Autodesk Inventor part; units mm, degrees
ref_plane "YZ Plane" through (0, 0, 0) normal (1, 0, 0) x (0, 1, 0)
ref_plane "XZ Plane" through (0, 0, 0) normal (0, 1, 0) x (-1, 0, 0)
ref_plane "XY Plane" through (0, 0, 0) normal (0, 0, 1) x (1, 0, 0)
sketch "Esquisse5" plane through (0, 0, 0) normal (0, 0, 1) x (1, 0, 0)
  line L0 (0, 0) -> (20, 0)
  line L1 (20, 0) -> (20, 30)
  line L2 (20, 30) -> (0, 30)
  line L3 (0, 30) -> (0, 0)
  line L4 (10, 0) -> (10, 30) construction
  circle A0 centre (10, 9) radius 2.15
  circle A1 centre (10, 15) radius 2.15
  circle A2 centre (10, 21) radius 2.15
  line L5 (10, 15) -> (20, 15) construction
  circle A3 centre (16, 15) radius 2.15
  circle A4 centre (4, 15) radius 2.15
  circle A5 centre (10, 15) radius 2.15
  dimension "d61" = 20
  dimension "d62" = 30
  dimension "d64" = 4.3
  dimension "d67" = 6
  dimension "d74" = 6
  dimension "d77" = 6
extrude "Extrusion5" add sketch "Esquisse5" along normal blind 2.2
sketch "Esquisse9" plane through (0, 0, 2.2) normal (0, 0, 1) x (1, 0, 0)
  line L0 (20, 0) -> (20, 30) construction
  line L1 (0, 30) -> (0, 0) construction
  line L2 (0, 30) -> (20, 30)
  line L3 (20, 30) -> (20, 27)
  line L4 (20, 27) -> (0, 27)
  line L5 (0, 27) -> (0, 30)
  line L6 (0, 15) -> (20, 15) construction
  line L7 (20, 0) -> (0, 0) construction
  line L8 (0, 0) -> (20, 0)
  line L9 (20, 0) -> (20, 3)
  line L10 (20, 3) -> (0, 3)
  line L11 (0, 3) -> (0, 0)
  dimension "d102" = 3
extrude "Extrusion9" add sketch "Esquisse9" along normal blind 10
sketch "Esquisse10" plane through (0, 0, 0) normal (0, -1, 0) x (1, 0, 0)
  line L0 (0, 0) -> (20, 0) construction
  line L1 (20, 0) -> (20, 12.2) construction
  line L2 (0, 12.2) -> (20, 12.2) construction
  line L3 (10, 12.2) -> (10, 0) construction
  circle A0 centre (10, 8.2) radius 2.15
  line L4 (10, 8.2) -> (20, 8.2) construction
  circle A1 centre (16, 8.2) radius 2.15
  circle A2 centre (4, 8.2) radius 2.15
  circle A3 centre (10, 8.2) radius 2.15
  dimension "d105" = 4
  dimension "d106" = 4.3
  dimension "d109" = 6
  dimension "d112" = 6
extrude "Extrusion10" cut sketch "Esquisse10" against normal through all
fillet "Congé6" radius 2 8 edges at (10, 0, 0) (10, 3, 2.2) (10, 27, 2.2) (0, 28.5, 12.2) (20, 28.5, 12.2) (20, 1.5, 12.2) (0, 1.5, 12.2) (10, 30, 0)
equation "\"d64\" = Holes"
equation "\"d80\" = Depth"
equation "\"d106\" = Holes"
equation "\"Depth\" = 2.2"
equation "\"Holes\" = 4.3"
equation "\"Height\" = 0"
equation "\"Rounding\" = 7"
properties part number "Pantilt"
Could you check a few things on this model? Use its own coordinates, in mm. A direction names the side the tool comes from. Give positions to 0.01 mm unless a question says otherwise; leave off trailing zeros. Loops run counter-clockwise (first coordinate to the right, second up) from the corner with the lowest first, then second, coordinate; pieces in that order, holes last. Notation, with made-up numbers: (-39, 69) -> (-18, 69) arc R27 cw to (-18, 95) -> close; hole circle Ø3 at (28.25, -23). An arc over 180 degrees is marked (long way). Return JSON: item names as keys, results as strings.
Item 1: If we section it at A-A on z = 8.2: Count the separate pieces of the cut face and the enclosed holes in it, plus the area to 3 significant figures.
Geometry results:
{"separate pieces": "8", "enclosed holes": "0", "area": "42.6 mm²"}
Item 2: We'd pull the mould along X, two halves only. Please class faces 3 (the cylindrical face through (1.85, 1.48, 8.29)), 4 (the flat face through (10, 29, 12.2)), 5 (the cylindrical face through (18.05, 1.48, 8.85)), 6 (the flat face through (20, 15, 2)): +X half, -X half, draft (parallel to the pull), parting line (faces both ways), or undercut.
Geometry results:
{"face 3": "undercut", "face 4": "draft", "face 5": "undercut", "face 6": "+X half"}
Item 3: If we section it at B-B on y = 9: List the corners of the cut face in (x, z) for me.
Geometry results:
{"outline": "(0, 0) -> (7.85, 0) -> (7.85, 2.2) -> (0, 2.2) -> close; (12.15, 0) -> (20, 0) -> (20, 2.2) -> (12.15, 2.2) -> close"}
Item 4: I need wall thicknesses on L1, parallel to X at y = 2.5, z = 8.75; L2, parallel to Y at x = 16.5, z = 11; L3, parallel to Z at x = 10, y = 2.25. Which ranges of each line are inside material? Lowest first, please. Write a range as from..to.
Geometry results:
{"L1": "x = 0..1.92, 6.08..7.92, 12.08..13.92, 18.08..20", "L2": "y = 0..3, 27..30", "L3": "z = 0..6.05, 10.35..12.2"}
Item 5: Which directions (+Z, -Z, +X, -X, +Y, -Y) give clear straight access to the entire face, cutting with the end or side of a thin tool? Please do faces 1 (the cylindrical face through (10.14, 0.57, 0.6)), 2 (the flat face through (12.4, 27, 8.1)).
Geometry results:
{"face 1": "-Z, +X, -X, -Y", "face 2": "+Z, +X, -X"}
Item 6: I'm going to push flat-ended pins straight in: pin 1 (4 mm diameter, centred on x = 16, z = 8.2, fed in from +Y); pin 2 (10 mm diameter, centred on x = 14.5, y = 17, fed in from +Z). Where does each tip first touch, or does it pass through?
Geometry results:
{"pin 1": "passes through", "pin 2": "stops at z = 2.2"}
Item 7: If we section it at D-D on x = 16: List the corners of the cut face in (y, z) for me, plus the area to 3 significant figures.
Geometry results:
{"outline": "(0, 2) arc R2 ccw to (2, 0) -> (12.85, 0) -> (12.85, 2.2) -> (5, 2.2) arc R2 cw to (3, 4.2) -> (3, 6.05) -> (0, 6.05) -> close; (0, 10.35) -> (3, 10.35) -> (3, 12.2) -> (0, 12.2) -> close; (17.15, 0) -> (28, 0) arc R2 ccw to (30, 2) -> (30, 6.05) -> (27, 6.05) -> (27, 4.2) arc R2 cw to (25, 2.2) -> (17.15, 2.2) -> close; (27, 10.35) -> (30, 10.35) -> (30, 12.2) -> (27, 12.2) -> close", "area": "90.7 mm²"}
